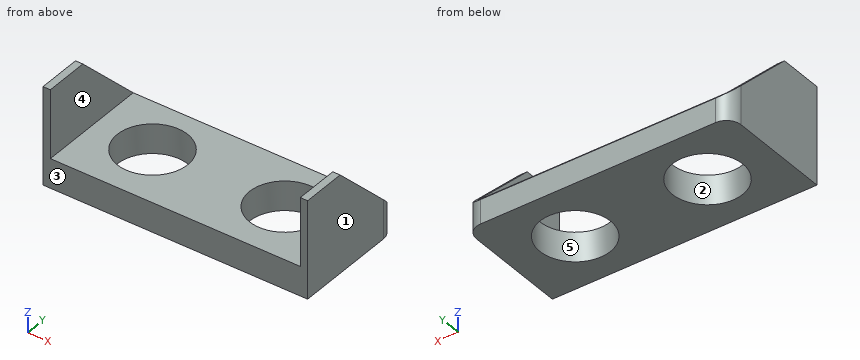
from build123d import *

# Parameters (mm, degrees)
BOSS_EXTRUDE1_DEPTH = 16
CHAMFER1_SIZE       = 10
FILLET1_R           = 2
SKETCH3_R           = 4.8
CUT_EXTRUDE1_DEPTH  = 42.57992304


with BuildPart() as part:
    # Sketch2 → Boss-Extrude1 (new body)
    with BuildSketch(Plane(origin=(0, 0, 0), x_dir=(1, 0, 0), z_dir=(0, 1, 0))):
        Polygon((0, 0), (0, 13.3), (36, 13.3), (36, 0), (35, 0), (35, 9.3), (1, 9.3), (1, 0), align=None)
    extrude(amount=BOSS_EXTRUDE1_DEPTH)

    # Chamfer1
    chamfer1_edges = [part.edges().sort_by_distance(p)[0] for p in [
        (0.5, 16, 0),
    ]]
    chamfer(chamfer1_edges, length=CHAMFER1_SIZE)

    # Fillet1
    fillet1_edges = [part.edges().sort_by_distance(p)[0] for p in [
        (36, 16, -11.65),
        (0, 16, -11.65),
    ]]
    fillet(fillet1_edges, radius=FILLET1_R)

    # Sketch3 → Cut-Extrude1 (cut, through all)
    with BuildSketch(Plane(origin=(0, 0, -13.3), x_dir=(-1, 0, 0), z_dir=(0, 0, -1))):
        with Locations((-27, 8)):
            Circle(SKETCH3_R)
        with Locations((-9, 8)):
            Circle(SKETCH3_R)
    extrude(amount=-CUT_EXTRUDE1_DEPTH, mode=Mode.SUBTRACT)


solid = part.part
Part model, mm, in its own coordinate system. Face numbers are marked on the shaded views. A direction names the side the tool comes from. Coordinates: 2 decimals unless noted, no trailing zeros. Loops run counter-clockwise (first coordinate to the right, second up) from the corner with the lowest first, then second, coordinate; pieces in that order, holes last. Notation, with made-up numbers: (-4, 16.25) -> (20, 16.25) arc R30 ccw to (20, 41.25) -> close; hole circle Ø10 at (47.25, -0.5). An arc over 180 degrees is marked (long way). Use a Markdown table: item, result. Add a question column.
Item 1: Band-saw the part on D-D on z = -4. Write the cut outline in (x, y).
Item 2: Band-saw the part on A-A on x = 27. Write the cut outline in (y, z).
Item 3: Flat gauge pin, fed straight in: P1, Ø2, axis at x = 6, y = 14, coming from the +Z side. Where does the tip first touch, or does it go through?
Item 4: Band-saw the part on C-C on z = -10.75. Write the cut outline in (x, y).
Item 5: Band-saw the part on B-B on y = 8. Write the cut outline in (x, z).
Item 6: Probe probe 1 along X at (y, z) = (5.5, -2); probe 2 along Y at (x, z) = (27, -11.45); probe 3 along X at (y, z) = (5, -9.75). List the from-to ranges inside material, lowest first.
Item 7: Pull direction Y, two halves, no side cores. Call the marked faces 1, 2 and 3: +Y half, -Y half, draft (parallel to the pull), parting line (faces both ways), or undercut.
Item 8: Which spindle directions (+Z, -Z, +X, -X, +Y, -Y) get a long thin tool onto all of the face, cutting with end or side? Do the marked faces 4 and 5. Say none if no direction does.
Geometry says:
| question | item | result |
|---|---|---|
| 1 | outline | (0, 0) -> (1, 0) -> (1, 10) -> (0, 10) -> close; (35, 0) -> (36, 0) -> (36, 10) -> (35, 10) -> close |
| 2 | outline | (0, -13.3) -> (3.2, -13.3) -> (3.2, -9.3) -> (0, -9.3) -> close; (12.8, -13.3) -> (16, -13.3) -> (16, -10) -> (15.3, -9.3) -> (12.8, -9.3) -> close |
| 3 | P1 | z = -9.3 |
| 4 | outline | (0, 0) -> (36, 0) -> (36, 14) arc R2 ccw to (34, 16) -> (2, 16) arc R2 ccw to (0, 14) -> close; hole circle Ø9.6 at (9, 8); hole circle Ø9.6 at (27, 8) |
| 5 | outline | (0, -13.3) -> (4.2, -13.3) -> (4.2, -9.3) -> (1, -9.3) -> (1, -2) -> (0, -2) -> close; (13.8, -13.3) -> (22.2, -13.3) -> (22.2, -9.3) -> (13.8, -9.3) -> close; (31.8, -13.3) -> (36, -13.3) -> (36, -2) -> (35, -2) -> (35, -9.3) -> (31.8, -9.3) -> close |
| 6 | probe 1 | 0 to 1, 35 to 36 |
| 6 | probe 2 | 0 to 3.2, 12.8 to 16 |
| 6 | probe 3 | 0 to 5.25, 12.75 to 23.25, 30.75 to 36 |
| 7 | face 1 | draft |
| 7 | face 2 | undercut |
| 7 | face 3 | -Y half |
| 8 | face 4 | +Z, +Y, -Y |
| 8 | face 5 | +Z, -Z |
